```python
from build123d import *

# Parameters (mm, degrees)
BOSS_EXTRUDE1_DEPTH = 5
D_GAGEMENT_M31_D    = 3.4
D_GAGEMENT_M32_D    = 3.4


with BuildPart() as part:
    # Sketch1 → Boss-Extrude1 (new body)
    with BuildSketch(Plane.XY):
        Polygon((10, -3.5), (20, -3.5), (20, -8.5), (-20, -8.5), (-20, -3.5), (-10, -3.5), (-10, 3.5), (10, 3.5), align=None)
    extrude(amount=BOSS_EXTRUDE1_DEPTH)

    # Dégagement M31 (through all)
    with Locations(Plane.XY.offset(5)):
        with Locations((3.580019281, -1.5), (-4.248289546, -1.5)):
            Hole(D_GAGEMENT_M31_D / 2)

    # Dégagement M32 (through all)
    with Locations(Plane(origin=(0, -3.5, 0), x_dir=(1, 0, 0), z_dir=(0, 1, 0))):
        with Locations((-15, -2.5), (15, -2.5)):
            Hole(D_GAGEMENT_M32_D / 2)


solid = part.part
```
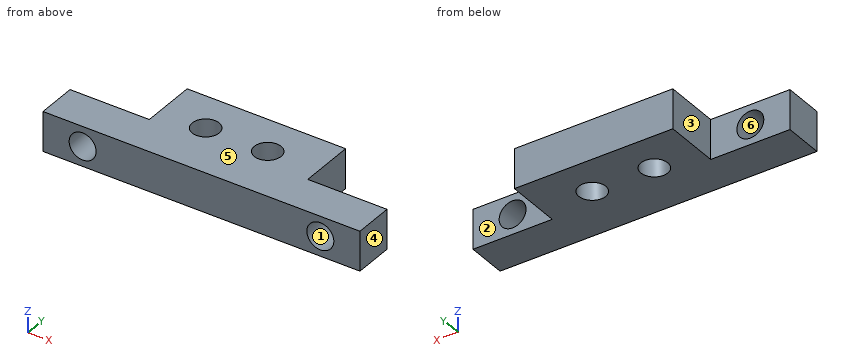
The model under review builds one solid part; all positions refer to its coordinate system, in mm. Face numbers are marked on the shaded views. A direction names the side the tool comes from. Round coordinates to 2 decimals unless told otherwise and drop trailing zeros. Loops run counter-clockwise (first coordinate to the right, second up) from the corner with the lowest first, then second, coordinate; pieces in that order, holes last. Notation, with made-up numbers: M -9,-10 L -2,-10 A26 ccw -2,5 Z; hole C 72,66 d5. An arc over 180 degrees is marked long. Write item = value, one per line.
Item 1: The part is to be moulded in two halves that separate along X. For the marked faces 4, 5 and 6, say which applies: released by +X, released by -X, zero draft, split by the parting line, or undercut.
Return value:
face_4 = released by +X
face_5 = zero draft
face_6 = undercut
Item 2: Machinability: for the marked faces 1, 2 and 3, which of the approach directions +Z, -Z, +X, -X, +Y, -Y give a long, thin tool a straight path to every point of the face, cutting with its end or side? Answer none if there is none.
Return value:
face_1 = +Y, -Y
face_2 = +Z, -Z, +X, +Y
face_3 = +Z, -Z, -X, +Y
Item 3: Take a section at B-B on x = -15. Write out the cut boundary in (y, z).
Return value:
outline = M -8.5,0 L -3.5,0 L -3.5,0.8 L -8.5,0.8 Z; M -8.5,4.2 L -3.5,4.2 L -3.5,5 L -8.5,5 Z
Item 4: Insertion check: P1, Ø2.5, axis at x = 3.58, y = -1.5, coming from the +Z side; P2, Ø1, axis at y = -1, z = 2, coming from the +X side. Each pin has a flat end and moves straight along its axis. Give the tip position at first contact, or say it passes through.
Return value:
P1 = through
P2 = 10
Item 5: Take a section at C-C on y = -1.5. Write out the cut boundary in (x, z), then the cut area to 3 significant figures.
Return value:
outline = M -10,0 L -5.95,0 L -5.95,5 L -10,5 Z; M -2.55,0 L 1.88,0 L 1.88,5 L -2.55,5 Z; M 5.28,0 L 10,0 L 10,5 L 5.28,5 Z
area = 66.0 mm2
Item 6: Take a section at A-A on z = 2.5. Write out the cut boundary in (x, y).
Return value:
outline = M -20,-8.5 L -16.7,-8.5 L -16.7,-3.5 L -20,-3.5 Z; M -13.3,-8.5 L 13.3,-8.5 L 13.3,-3.5 L 10,-3.5 L 10,3.5 L -10,3.5 L -10,-3.5 L -13.3,-3.5 Z; M 16.7,-8.5 L 20,-8.5 L 20,-3.5 L 16.7,-3.5 Z; hole C -4.25,-1.5 d3.4; hole C 3.58,-1.5 d3.4
Item 7: For line 1 (X direction, y = -5.75, z = 1.65); line 2 (X direction, y = -1, z = 0.25); line 3 (Z direction, x = 15, y = -5.4), list the stretches that pass through material, from the lowest coordinate up. Write a range as [from, to].
Return value:
line_1 = [-20, -16.47], [-13.53, 13.53], [16.47, 20]
line_2 = [-10, -5.87], [-2.62, 1.96], [5.2, 10]
line_3 = [0, 0.8], [4.2, 5]
Item 8: Take a section at D-D on y = 2.75. Write out the cut boundary in (x, z).
Return value:
outline = M -10,0 L 10,0 L 10,5 L -10,5 Z
